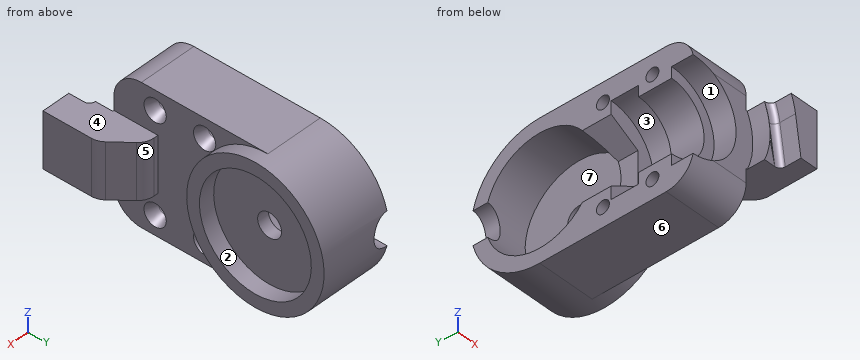
from build123d import *
from build123d.topology import SkipClean

# Parameters (mm, degrees)
CROQUIS1_W                       = 10.5
CROQUIS1_H                       = 25
SALIENTE_EXTRUIR1_DEPTH          = 28
CROQUIS2_R                       = 12.5
SALIENTE_EXTRUIR2_DEPTH          = 13
REDONDEO1_START                  = -1
REDONDEO1_DEPTH                  = 12
CORTAR_EXTRUIR1_DEPTH            = 13
CROQUIS5_R                       = 9.915
CORTAR_EXTRUIR2_DEPTH            = 8
CROQUIS8_R                       = 1.175
CORTAR_EXTRUIR5_DEPTH            = 50.338119296
CROQUIS10_W                      = 6.5
CROQUIS10_H                      = 15
SALIENTE_EXTRUIR3_DEPTH          = 5
CORTAR_EXTRUIR6_DEPTH            = 7
CORTAR_EXTRUIR7_DEPTH            = 3.85
CHAFL_N1_SIZE                    = 4.3
CHAFL_N1_SIZE2                   = 5.124540448
REDONDEO2_R                      = 1
REDONDEO3_R                      = 3
CORTAR_EXTRUIR8_START            = -2.5
CORTAR_EXTRUIR8_DEPTH            = 2.5
CROQUIS14_R                      = 3.6
CORTAR_EXTRUIR9_DEPTH            = 49.739101502
CROQUIS15_R                      = 2.025
CORTAR_EXTRUIR10_DEPTH           = 2
CORTAR_EXTRUIR10_DRAFT           = -23
CORTAR_EXTRUIR10_PROFILE_2_DEPTH = 2
CORTAR_EXTRUIR10_PROFILE_2_DRAFT = -23
CORTAR_EXTRUIR10_PROFILE_3_DEPTH = 2
CORTAR_EXTRUIR10_PROFILE_3_DRAFT = -23
CORTAR_EXTRUIR10_PROFILE_4_DEPTH = 2
CORTAR_EXTRUIR10_PROFILE_4_DRAFT = -23
CROQUIS16_R                      = 3.6
SALIENTE_EXTRUIR4_DEPTH          = 2.5
CROQUIS17_R                      = 12.5
SALIENTE_EXTRUIR5_DEPTH          = 2.5
CROQUIS18_R                      = 2.175
CORTAR_EXTRUIR11_DEPTH           = 50.338119296
CROQUIS19_R                      = 10.175
CORTAR_EXTRUIR12_DEPTH           = 2.85


with BuildPart() as part:
    # Croquis1 → Saliente-Extruir1 (new body)
    with BuildSketch(Plane(origin=(0, 0, 0), x_dir=(1, 0, 0), z_dir=(0, 1, 0))):
        with Locations((5.25, 12.5)):
            Rectangle(CROQUIS1_W, CROQUIS1_H)
    extrude(amount=SALIENTE_EXTRUIR1_DEPTH)

    # Croquis2 → Saliente-Extruir2 (add)
    with BuildSketch(Plane.ZY):
        with Locations((-12.5, 28)):
            Circle(CROQUIS2_R)
    extrude(amount=-SALIENTE_EXTRUIR2_DEPTH)

    # Croquis3 → Cortar-Revolución1 (revolve, cut)
    with BuildSketch(Plane.ZY):
        Polygon((-4, 0.5), (-4, 4), (-6, 4), (-6, 10), (-4, 10), (-4, 15), (-9.5, 15), (-9.5, 41), (-12.5, 41), (-12.5, 0), (-4, 0), align=None)
    revolve(axis=Axis((0, 0, -12.5), (0, 1, 0)), mode=Mode.SUBTRACT)

    # Redondeo1: read off the stored shape, not the designer's step
    # Redondeo1 outline → Redondeo1 (cut)
    with BuildSketch(Plane.YZ.offset(REDONDEO1_START)):
        with BuildLine():
            Line((0, 0), (0, -5))
            ThreePointArc((0, -5), (1.464466094, -1.464466094), (5, 0))
            Line((5, 0), (0, 0))
        make_face()
        with BuildLine():
            ThreePointArc((5, -25), (1.464466094, -23.535533906), (0, -20))
            Line((0, -20), (0, -25))
            Line((0, -25), (5, -25))
        make_face()
    extrude(amount=REDONDEO1_DEPTH, mode=Mode.SUBTRACT)

    # Croquis4 → Cortar-Extruir1 (cut)
    with BuildSketch(Plane.XZ.offset(-15)):
        Polygon((0, -18.67764788), (5.35, -15.58882394), (5.35, -9.41117606), (0, -6.32235212), (-5.35, -9.41117606), (-5.35, -15.58882394), align=None)
    extrude(amount=-CORTAR_EXTRUIR1_DEPTH, mode=Mode.SUBTRACT)

    # Croquis5 → Cortar-Extruir2 (cut)
    with BuildSketch(Plane.ZY):
        with Locations((-12.5, 28)):
            Circle(CROQUIS5_R)
    extrude(amount=-CORTAR_EXTRUIR2_DEPTH, mode=Mode.SUBTRACT)

    # Croquis8 → Cortar-Extruir5 (cut, through all)
    with BuildSketch(Plane.ZY):
        with Locations((-21.5, 16.5)):
            Circle(CROQUIS8_R)
        with Locations((-3.5, 16.5)):
            Circle(CROQUIS8_R)
        with Locations((-3.5, 7.5)):
            Circle(CROQUIS8_R)
        with Locations((-21.5, 7.5)):
            Circle(CROQUIS8_R)
    extrude(amount=-CORTAR_EXTRUIR5_DEPTH, mode=Mode.SUBTRACT)

    # Croquis10 → Saliente-Extruir3 (add, symmetric)
    with BuildSketch(Plane.XY.offset(-12.5)):
        with Locations((13.75, 0.5)):
            Rectangle(CROQUIS10_W, CROQUIS10_H)
    extrude(amount=SALIENTE_EXTRUIR3_DEPTH, both=True)

    # Croquis11 → Cortar-Extruir6 (cut)
    with BuildSketch(Plane.XZ.offset(7)):
        with BuildLine():
            Line((10.5, -17.5), (10.743486399, -17.5))
            ThreePointArc((10.743486399, -17.5), (11.85, -12.5), (10.743486399, -7.5))
            Line((10.743486399, -7.5), (10.5, -7.5))
            Line((10.5, -7.5), (10.5, -17.5))
        make_face()
    extrude(amount=-CORTAR_EXTRUIR6_DEPTH, mode=Mode.SUBTRACT)

    # Croquis12 → Cortar-Extruir7 (cut)
    with BuildSketch(Plane.XZ.offset(7)):
        with BuildLine():
            ThreePointArc((10.743486399, -7.5), (11.85, -12.5), (10.743486399, -17.5))
            Line((10.743486399, -17.5), (13.787722048, -17.5))
            Line((13.787722048, -17.5), (12.6958, -10.515267686))
            ThreePointArc((12.6958, -10.515267686), (12.358868803, -8.981355103), (11.837335004, -7.5))
            Line((11.837335004, -7.5), (10.743486399, -7.5))
        make_face()
    extrude(amount=-CORTAR_EXTRUIR7_DEPTH, mode=Mode.SUBTRACT)

    # Chaflán1
    chafl_n1_edges = [part.edges().sort_by_distance(p)[0] for p in [
        (17, 8, -12.5),
    ]]
    chafl_n1_side = [part.faces().sort_by_distance(p)[0] for p in [
        (13.75, 8, -12.5),
    ]]
    chamfer(chafl_n1_edges, length=CHAFL_N1_SIZE, length2=CHAFL_N1_SIZE2, reference=chafl_n1_side[0])

    # Redondeo2
    redondeo2_edges = [part.edges().sort_by_distance(p)[0] for p in [
        (12.358868803, -3.15, -8.981355103),
        (13.241761024, -3.15, -14.007633843),
    ]]
    fillet(redondeo2_edges, radius=REDONDEO2_R - 0.0001)  # a hair under: the kernel refuses the full size

    # Redondeo3
    redondeo3_edges = [part.edges().sort_by_distance(p)[0] for p in [
        (12.7, 8, -12.5),
        (17, 2.875459552, -12.5),
    ]]
    fillet(redondeo3_edges, radius=REDONDEO3_R)

    # Croquis13 → Cortar-Extruir8 (cut)
    with BuildSketch(Plane(origin=(13, 0, 0), x_dir=(0, 0, -1), z_dir=(1, 0, 0)).offset(CORTAR_EXTRUIR8_START)):
        with BuildLine():
            ThreePointArc((9.860236176, 30.44778409), (8.9, 28), (9.860236176, 25.55221591))
            Line((9.860236176, 25.55221591), (10.393008213, 15.678856157))
            ThreePointArc((10.393008213, 15.678856157), (12.51082596, 15.500004688), (14.628330733, 15.682524273))
            Line((14.628330733, 15.682524273), (15.272384177, 25.703505721))
            ThreePointArc((15.272384177, 25.703505721), (16.1, 28), (15.272384177, 30.296494279))
            Line((15.272384177, 30.296494279), (14.628330733, 40.317475727))
            ThreePointArc((14.628330733, 40.317475727), (12.51082596, 40.499995312), (10.393008213, 40.321143843))
            Line((10.393008213, 40.321143843), (9.860236176, 30.44778409))
        make_face()
    extrude(amount=CORTAR_EXTRUIR8_DEPTH, mode=Mode.SUBTRACT)

    # Croquis14 → Cortar-Extruir9 (cut, through all)
    with SkipClean():  # the faces are left unmerged after this step: merging them gives an invalid solid
        with BuildSketch(Plane(origin=(10.5, 0, 0), x_dir=(0, 0, -1), z_dir=(1, 0, 0))):
            with Locations(Location((12.5, 28, 0), (0, 0, 39.636527191))):
                Circle(CROQUIS14_R)
        extrude(amount=-CORTAR_EXTRUIR9_DEPTH, mode=Mode.SUBTRACT)


with BuildPart() as cortar_extruir10_tool:
    # Croquis15 → Cortar-Extruir10 (with draft: the straight prism first)
    with BuildSketch(Plane(origin=(10.5, 0, 0), x_dir=(0, 0, -1), z_dir=(1, 0, 0))):
        with Locations((3.5, 16.5)):
            Circle(CROQUIS15_R)
    extrude(amount=-CORTAR_EXTRUIR10_DEPTH)
    # Cortar-Extruir10: the draft: its side faces are tilted about the plane it starts from
    cortar_extruir10_sides = [cortar_extruir10_tool.faces().sort_by_distance(p)[0] for p in [
        (9.5, 16.5, -1.475),
    ]]
    draft(cortar_extruir10_sides, Plane(origin=(10.5, 0, 0), x_dir=(0, 0, -1), z_dir=(1, 0, 0)), CORTAR_EXTRUIR10_DRAFT)


with BuildPart() as part_1:
    add(part.part)

    # Cortar-Extruir10: cut by cortar_extruir10_tool
    add(cortar_extruir10_tool.part, mode=Mode.SUBTRACT)


with BuildPart() as cortar_extruir10_profile_2_tool:
    # Croquis15 → Cortar-Extruir10 profile 2 (with draft: the straight prism first)
    with BuildSketch(Plane(origin=(10.5, 0, 0), x_dir=(0, 0, -1), z_dir=(1, 0, 0))):
        with Locations((3.5, 7.5)):
            Circle(CROQUIS15_R)
    extrude(amount=-CORTAR_EXTRUIR10_PROFILE_2_DEPTH)
    # Cortar-Extruir10 profile 2: the draft: its side faces are tilted about the plane it starts from
    cortar_extruir10_profile_2_sides = [cortar_extruir10_profile_2_tool.faces().sort_by_distance(p)[0] for p in [
        (9.5, 7.5, -1.475),
    ]]
    draft(cortar_extruir10_profile_2_sides, Plane(origin=(10.5, 0, 0), x_dir=(0, 0, -1), z_dir=(1, 0, 0)), CORTAR_EXTRUIR10_PROFILE_2_DRAFT)


with BuildPart() as part_2:
    add(part_1.part)

    # Cortar-Extruir10 profile 2: cut by cortar_extruir10_profile_2_tool
    add(cortar_extruir10_profile_2_tool.part, mode=Mode.SUBTRACT)


with BuildPart() as cortar_extruir10_profile_3_tool:
    # Croquis15 → Cortar-Extruir10 profile 3 (with draft: the straight prism first)
    with BuildSketch(Plane(origin=(10.5, 0, 0), x_dir=(0, 0, -1), z_dir=(1, 0, 0))):
        with Locations((21.5, 7.5)):
            Circle(CROQUIS15_R)
    extrude(amount=-CORTAR_EXTRUIR10_PROFILE_3_DEPTH)
    # Cortar-Extruir10 profile 3: the draft: its side faces are tilted about the plane it starts from
    cortar_extruir10_profile_3_sides = [cortar_extruir10_profile_3_tool.faces().sort_by_distance(p)[0] for p in [
        (9.5, 7.5, -19.475),
    ]]
    draft(cortar_extruir10_profile_3_sides, Plane(origin=(10.5, 0, 0), x_dir=(0, 0, -1), z_dir=(1, 0, 0)), CORTAR_EXTRUIR10_PROFILE_3_DRAFT)


with BuildPart() as part_3:
    add(part_2.part)

    # Cortar-Extruir10 profile 3: cut by cortar_extruir10_profile_3_tool
    add(cortar_extruir10_profile_3_tool.part, mode=Mode.SUBTRACT)


with BuildPart() as cortar_extruir10_profile_4_tool:
    # Croquis15 → Cortar-Extruir10 profile 4 (with draft: the straight prism first)
    with BuildSketch(Plane(origin=(10.5, 0, 0), x_dir=(0, 0, -1), z_dir=(1, 0, 0))):
        with Locations((21.5, 16.5)):
            Circle(CROQUIS15_R)
    extrude(amount=-CORTAR_EXTRUIR10_PROFILE_4_DEPTH)
    # Cortar-Extruir10 profile 4: the draft: its side faces are tilted about the plane it starts from
    cortar_extruir10_profile_4_sides = [cortar_extruir10_profile_4_tool.faces().sort_by_distance(p)[0] for p in [
        (9.5, 16.5, -19.475),
    ]]
    draft(cortar_extruir10_profile_4_sides, Plane(origin=(10.5, 0, 0), x_dir=(0, 0, -1), z_dir=(1, 0, 0)), CORTAR_EXTRUIR10_PROFILE_4_DRAFT)


with BuildPart() as part_4:
    add(part_3.part)

    # Cortar-Extruir10 profile 4: cut by cortar_extruir10_profile_4_tool
    add(cortar_extruir10_profile_4_tool.part, mode=Mode.SUBTRACT)

    # Croquis16 → Saliente-Extruir4 (add)
    with BuildSketch(Plane.ZY.offset(-8)):
        with Locations((-12.5, 28)):
            Circle(CROQUIS16_R)
    extrude(amount=-SALIENTE_EXTRUIR4_DEPTH)

    # Croquis17 → Saliente-Extruir5 (add)
    with BuildSketch(Plane(origin=(10.5, 0, 0), x_dir=(0, 0, -1), z_dir=(1, 0, 0))):
        with Locations(Location((12.5, 28, 0), (0, 0, 180))):
            Circle(CROQUIS17_R)
    extrude(amount=SALIENTE_EXTRUIR5_DEPTH)

    # Croquis18 → Cortar-Extruir11 (cut, through all)
    with BuildSketch(Plane(origin=(13, 0, 0), x_dir=(0, 0, -1), z_dir=(1, 0, 0))):
        with Locations((12.5, 28)):
            Circle(CROQUIS18_R)
    extrude(amount=-CORTAR_EXTRUIR11_DEPTH, mode=Mode.SUBTRACT)

    # Croquis19 → Cortar-Extruir12 (cut)
    with BuildSketch(Plane(origin=(13, 0, 0), x_dir=(0, 0, -1), z_dir=(1, 0, 0))):
        with Locations((12.5, 28)):
            Circle(CROQUIS19_R)
    extrude(amount=-CORTAR_EXTRUIR12_DEPTH, mode=Mode.SUBTRACT)


solid = part_4.part
For this review, take the finished solid that the model builds, in its own axes (mm). Face numbers are marked on the shaded views. A direction names the side the tool comes from. Round coordinates to 2 decimals unless told otherwise and drop trailing zeros. Write each loop counter-clockwise with the first axis right and the second up, starting at its lowest first coordinate (ties: lowest second). Pieces come first, ordered by that corner, then holes. Notation, with made-up numbers: (46, -29.75) - (63, -29.75) arc R29 cw to (63, 0.25) - close; hole circle Ø7 at (56, 2). An arc over 180 degrees is marked (long way). Use a Markdown table: item, result.
Q1. Wall thickness on line 1 along Y through (x, z) = (8.95, -12.5) (3 decimals); line 2 along Z through (x, y) = (6.75, 28) (3 decimals); line 3 along Y through (x, z) = (5.75, -18.25): over which ranges is each line inside the solid? List them lowest first.
Derived:
| item | result |
|---|---|
| line 1 | y = 0 to 25.825, 30.175 to 40.5 |
| line 2 | z = -25 to -22.415, -2.585 to 0 |
| line 3 | y = 4 to 10, 15 to 19.92, 36.08 to 39.1 |
Q2. We need section D-D (x = 4.5). Give the boundary of the cut face in (y, z) (3 decimals).
Derived:
| item | result |
|---|---|
| outline | (0, -20) arc R5 ccw to (5, -25) - (28, -25) arc R12.5 ccw to (28, 0) - (5, 0) arc R5 ccw to (0, -5) - (0, -5.289) - (4, -5.289) - (4, -7.81) - (10, -7.81) - (10, -5.289) - (15, -5.289) - (15, -8.92) - (18.754, -8.92) arc R9.915 cw (long way) to (18.754, -16.08) - (15, -16.08) - (15, -19.711) - (10, -19.711) - (10, -17.19) - (4, -17.19) - (4, -19.711) - (0, -19.711) - close; hole circle Ø2.35 at (7.5, -21.5); hole circle Ø2.35 at (7.5, -3.5); hole circle Ø2.35 at (16.5, -21.5); hole circle Ø2.35 at (16.5, -3.5) |
Q3. Machinability: for the marked faces 1, 2, 3 and 4, which of the approach directions +Z, -Z, +X, -X, +Y, -Y give a long, thin tool a straight path to every point of the face, cutting with its end or side? Answer none if there is none.
Derived:
| item | result |
|---|---|
| face 1 | -X, -Y |
| face 2 | +X |
| face 3 | -X |
| face 4 | +Z, +X, -Y |
Q4. We need section C-C (y = 11.5). Give the boundary of the cut face in (x, z).
Derived:
| item | result |
|---|---|
| outline | (0, -25) - (10.5, -25) - (10.5, 0) - (0, 0) - (0, -4) arc R8.5 cw to (0, -21) - close |
Q5. We need section A-A (z = -3.5). State how many separate pieces and enclosed holes the cut face has, plus the area to 3 significant figures.
Derived:
| item | result |
|---|---|
| separate pieces | 3 |
| enclosed holes | 0 |
| area | 280 mm2 |
Q6. Clearance check with flat-ended pins moving along their axes: pin 1 (7 mm diameter, centred on x = 14, y = -1.5, fed in from -Z); pin 2 (4 mm diameter, centred on x = 11.5, y = 1, fed in from -Z); pin 3 (1.5 mm diameter, centred on y = 31.5, z = -12, fed in from -X). State where each tip first meets the part, or that it passes through.
Derived:
| item | result |
|---|---|
| pin 1 | stops at z = -17.5 |
| pin 2 | stops at z = -24.46 |
| pin 3 | stops at x = 8 |
Q7. The part is to be moulded in two halves that separate along Z. For the marked faces 5, 6 and 7, say which applies: pulls with the +Z half, pulls with the -Z half, needs draft (parallel to the pull), parting line crosses it, or undercut.
Derived:
| item | result |
|---|---|
| face 5 | needs draft |
| face 6 | pulls with the -Z half |
| face 7 | undercut |
